For this review, use the dimensioned drawing (mm, ordinates from the lowest corner) and the shaded views. A direction names the side the tool comes from. Coordinates: 2 decimals unless noted, no trailing zeros. Loops run counter-clockwise (first coordinate to the right, second up) from the corner with the lowest first, then second, coordinate; pieces in that order, holes last. Notation, with made-up numbers: M -18,31.5 L -3,31.5 A11 ccw -3,38.5 Z; hole C 56.25,83 d7. An arc over 180 degrees is marked long. One line per item, written item: value.
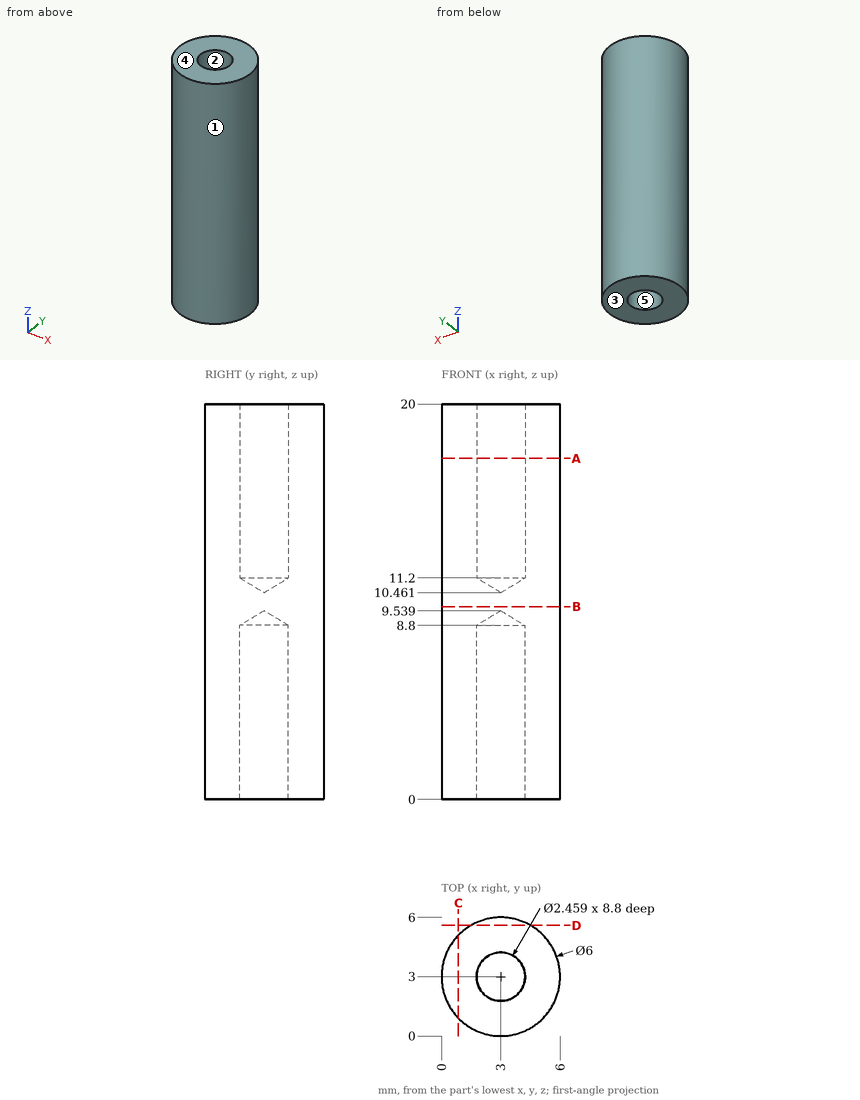
(1) Draft analysis for pull direction X (two halves, no side actions). For the marked faces 1, 2 and 3, state which applies: pulls with the +X half, pulls with the -X half, needs draft (parallel to the pull), parting line crosses it, or undercut.
Checks:
face 1: parting line crosses it
face 2: undercut
face 3: needs draft
(2) Add section C-C on x = 0.85. State the section outline as (y, z) points.
Checks:
outline: M 0.91,0 L 5.09,0 L 5.09,20 L 0.91,20 Z
(3) Insertion check: pin 1 Ø2 at (x, y) = (3, 3) entering from +Z; pin 2 Ø1 at (x, z) = (0.5, 13) entering from +Y; pin 3 Ø3 at (x, z) = (1, 10.5) entering from +Y. Each pin has a flat end and moves straight along its axis. Give the tip position at first contact, or say it passes through.
Checks:
pin 1: z = 11.06
pin 2: y = 5.24
pin 3: y = 5.96
(4) Add section B-B on z = 9.75. State the section outline as (x, y) points, then the cut area to 3 significant figures.
Checks:
outline: C 3,3 d6
area: 28.3 mm^2
(5) Add section A-A on z = 17.25. State the section outline as (x, y) points.
Checks:
outline: C 3,3 d6; hole C 3,3 d2.46
(6) Add section D-D on y = 5.6. State the section outline as (x, z) points.
Checks:
outline: M 1.5,0 L 4.5,0 L 4.5,20 L 1.5,20 Z
(7) To check wall thickness, follow L1, parallel to Y at x = 3, z = 17.5; L2, parallel to X at y = 2, z = 11.25 (1 decimal); L3, parallel to Y at x = 2.25, z = 16.25 (1 decimal). State the ranges of each line that lie inside material, in increasing order. Write a range as [from, to].
Checks:
L1: [0, 1.77], [4.23, 6]
L2: [0.2, 2.3], [3.7, 5.8]
L3: [0.1, 2], [4, 5.9]
(8) Tool access review of the marked faces 4 and 5: name each direction out of +Z, -Z, +X, -X, +Y, -Y from which nothing blocks a thin tool from reaching the whole face with its end or side.
Checks:
face 4: +Z, +X, -X, +Y, -Y
face 5: -Z
